Part print with two shaded views. Sizes in mm from the minimum x, y, z corner. Round coordinates to 2 decimals unless told otherwise and drop trailing zeros. Write each loop counter-clockwise with the first axis right and the second up, starting at its lowest first coordinate (ties: lowest second). Pieces come first, ordered by that corner, then holes. Notation, with made-up numbers: (28.5, 35) -> (35.5, 35) arc R35 cw to (35.5, 72) -> close; hole circle Ø8 at (23.5, -2). An arc over 180 degrees is marked (long way). Put each result on its own line as item: value. Start each with the question number.
1. Saw through at B-B on z = 6. List the corners of the cut face in (x, y), and give its area (3 significant figures).
2. Saw through at A-A on x = 5. List the corners of the cut face in (y, z).
3. Flat gauge pins, fed straight in: P1, Ø2, axis at x = 6.5, y = 3, coming from the +Z side; P2, Ø1.5, axis at x = 6, y = 3.5, coming from the +Z side (1 decimal); P3, Ø1.5, axis at x = 7, y = 1.5, coming from the -Z side; P4, Ø2, axis at x = 3.5, z = 3.5, coming from the +Y side. Where does each tip first touch, or does it go through?
4. Saw through at C-C on y = 0.7. List the corners of the cut face in (x, z).
5. Drill centre lines: line 1 (X direction, y = 3.8, z = 4.5); line 2 (Z direction, x = 3, y = 3.2); line 3 (X direction, y = 1.45, z = 6) (1 decimal). Where is each one in solid material? Low to high. Write a range as from..to.
6. Saw through at D-D on z = 8.5. List the corners of the cut face in (x, y), and give its area (3 significant figures).
7. Pull direction Z, two halves, no side cores. Call the marked faces 1, 2 and 3: pulls with the +Z half, pulls with the -Z half, needs draft (parallel to the pull), parting line crosses it, or undercut.
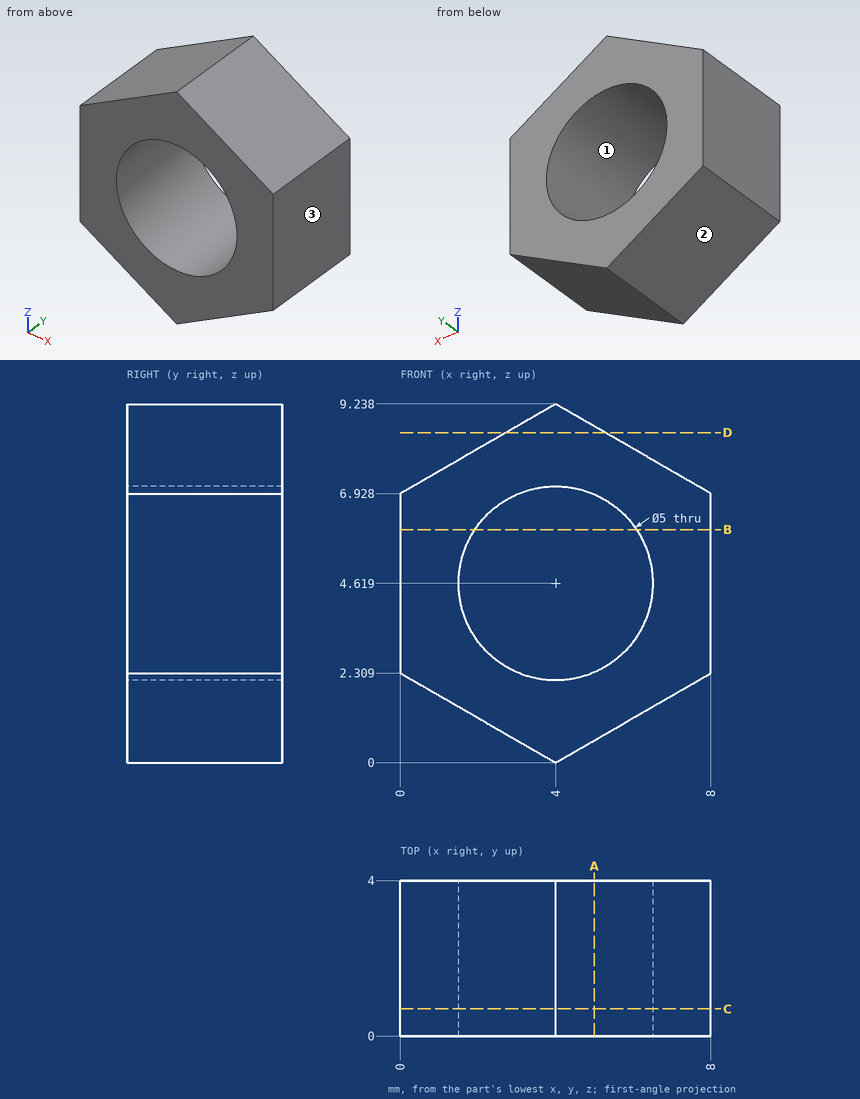
Return value:
1. outline: (0, 0) -> (1.92, 0) -> (1.92, 4) -> (0, 4) -> close; (6.08, 0) -> (8, 0) -> (8, 4) -> (6.08, 4) -> close
1. area: 15.3 mm^2
2. outline: (0, 0.58) -> (4, 0.58) -> (4, 2.33) -> (0, 2.33) -> close; (0, 6.91) -> (4, 6.91) -> (4, 8.66) -> (0, 8.66) -> close
3. P1: stops at z = 8.37
3. P2: stops at z = 8.5
3. P3: stops at z = 1.3
3. P4: passes through
4. outline: (0, 2.31) -> (4, 0) -> (8, 2.31) -> (8, 6.93) -> (4, 9.24) -> (0, 6.93) -> close; hole circle Ø5 at (4, 4.62)
5. line 1: x = 0..1.5, 6.5..8
5. line 2: z = 0.58..2.33, 6.91..8.66
5. line 3: x = 0..1.9, 6.1..8
6. outline: (2.72, 0) -> (5.28, 0) -> (5.28, 4) -> (2.72, 4) -> close
6. area: 10.2 mm^2
7. face 1: undercut
7. face 2: pulls with the -Z half
7. face 3: needs draft
